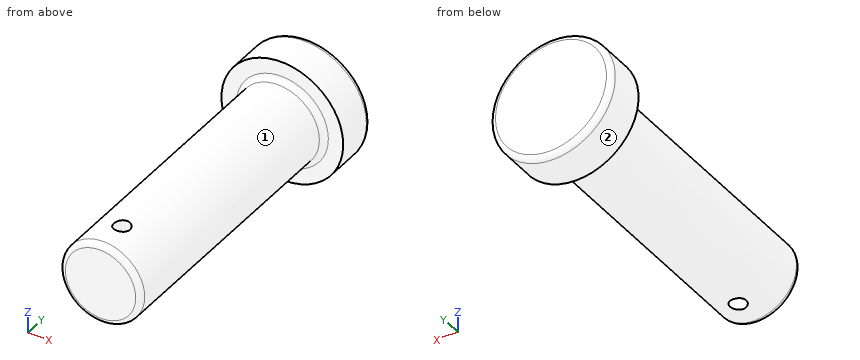
from build123d import *

# Parameters (mm, degrees)
SKETCH1_R               = 22.5
BOSS_EXTRUDE1_DEPTH     = 15
SKETCH2_R               = 15
BOSS_EXTRUDE2_DEPTH     = 102
FILLET1_R               = 2
SKETCH3_R               = 3
CUT_EXTRUDE1_DEPTH      = 23.5
CUT_EXTRUDE1_DEPTH_BACK = 23.5


with BuildPart() as part:
    # Sketch1 → Boss-Extrude1 (new body)
    with BuildSketch(Plane(origin=(0, 0, 0), x_dir=(1, 0, 0), z_dir=(0, 1, 0))):
        Circle(SKETCH1_R)
    extrude(amount=BOSS_EXTRUDE1_DEPTH)

    # Sketch2 → Boss-Extrude2 (add)
    with BuildSketch(Plane.XZ):
        Circle(SKETCH2_R)
    extrude(amount=BOSS_EXTRUDE2_DEPTH)

    # Fillet1
    fillet1_edges = [part.edges().sort_by_distance(p)[0] for p in [
        (-22.5, 15, 0),
        (-15, 0, 0),
        (-15, -102, 0),
    ]]
    fillet(fillet1_edges, radius=FILLET1_R)

    # Sketch3 → Cut-Extrude1 (cut, two sides)
    with BuildSketch(Plane.XY) as cut_extrude1_sk:
        with Locations((0, -90)):
            Circle(SKETCH3_R)
    extrude(amount=CUT_EXTRUDE1_DEPTH, mode=Mode.SUBTRACT)
    extrude(cut_extrude1_sk.sketch, amount=-CUT_EXTRUDE1_DEPTH_BACK, mode=Mode.SUBTRACT)


solid = part.part
Source: CAD feature listing. Evaluate the final solid. Frame: model axes, mm. Face numbers are marked on the shaded views. A direction names the side the tool comes from. Coordinates: 2 decimals unless noted, no trailing zeros. Loops run counter-clockwise (first coordinate to the right, second up) from the corner with the lowest first, then second, coordinate; pieces in that order, holes last. Notation, with made-up numbers: (78, 64.25) -> (87, 64.25) arc R3 ccw to (87, 69.25) -> close; hole circle Ø8 at (19.5, 32). An arc over 180 degrees is marked (long way). Answer in a Markdown table with one row per item. Add a question column.
Q1. Section D-D on y = -90. Return the cut outline in (x, z).
Q2. Contact query for flat-ended pins moving along their axis: pin 1 Ø1.5 at (x, y) = (-11.5, -74.5) entering from -Z; pin 2 Ø5 at (x, y) = (-5.5, -23.5) entering from -Z; pin 3 Ø5 at (x, y) = (0, -90) entering from +Z; pin 4 Ø3 at (x, z) = (-18, -6) entering from -Y. Output: stop coordinate, or through.
Q3. Reachability of the marked faces 1 and 2 from +Z, -Z, +X, -X, +Y, -Y: full face, straight path, thin tool, end or side. Return the list, or none.
Q4. Ray query, line 1 along X through (y, z) = (-90, 0.5); line 2 along Y through (x, z) = (0, -2); line 3 along X through (y, z) = (-90, -5). Return the intervals inside material, ascending.
Q5. Section A-A on x = 0. Return the cut outline in (y, z).
Q6. Section B-B on z = 0. Return the cut outline in (x, y), and give its area (4 significant figures).
Q7. Section C-C on y = -23. Return the cut outline in (x, z), and give its area (3 significant figures).
Computed values:
| question | item | result |
|---|---|---|
| 1 | outline | (-3, -14.7) -> (-3, 14.7) arc R15 ccw to start; (3, -14.7) arc R15 ccw to (3, 14.7) -> close |
| 2 | pin 1 | stops at z = -10.46 |
| 2 | pin 2 | stops at z = -14.7 |
| 2 | pin 3 | passes through |
| 2 | pin 4 | stops at y = 0 |
| 3 | face 1 | -Y |
| 3 | face 2 | +Y, -Y |
| 4 | line 1 | x = -14.99 to -3, 3 to 14.99 |
| 4 | line 2 | y = -102 to -93, -87 to 15 |
| 4 | line 3 | x = -14.14 to -3, 3 to 14.14 |
| 5 | outline | (-102, -13) arc R2 ccw to (-100, -15) -> (-93, -15) -> (-93, 15) -> (-100, 15) arc R2 ccw to (-102, 13) -> close; (-87, -15) -> (-2, -15) arc R2 cw to (0, -17) -> (0, -22.5) -> (13, -22.5) arc R2 ccw to (15, -20.5) -> (15, 20.5) arc R2 ccw to (13, 22.5) -> (0, 22.5) -> (0, 17) arc R2 cw to (-2, 15) -> (-87, 15) -> close |
| 6 | outline | (-22.5, 0) -> (-17, 0) arc R2 cw to (-15, -2) -> (-15, -100) arc R2 ccw to (-13, -102) -> (13, -102) arc R2 ccw to (15, -100) -> (15, -2) arc R2 cw to (17, 0) -> (22.5, 0) -> (22.5, 13) arc R2 ccw to (20.5, 15) -> (-20.5, 15) arc R2 ccw to (-22.5, 13) -> close; hole circle Ø6 at (0, -90) |
| 6 | area | 3,705 mm^2 |
| 7 | outline | circle Ø30 at (0, 0) |
| 7 | area | 707 mm^2 |
